Autodesk Inventor part; units mm, degrees
ref_plane "YZ Plane" through (0, 0, 0) normal (1, 0, 0) x (0, 1, 0)
ref_plane "XZ Plane" through (0, 0, 0) normal (0, 1, 0) x (-1, 0, 0)
ref_plane "XY Plane" through (0, 0, 0) normal (0, 0, 1) x (1, 0, 0)
sketch "Sketch1" plane through (0, 0, 0) normal (0, 0, 1) x (1, 0, 0)
  line L0 (0, 4.0132) -> (0, -0.9652)
  line L1 (-1.524, 0) -> (9.144, 0)
  line L2 (7.62, 0) -> (0, 0)
  line L3 (0, 0) -> (0, 0.762)
  line L4 (0, 0.762) -> (7.62, 0.762)
  line L5 (7.62, 0.762) -> (7.62, 0)
  line L6 (0, 0.762) -> (0.762, 0.762)
  line L7 (0.762, 0.762) -> (0.762, 3.302)
  line L8 (0.762, 3.302) -> (0, 3.302)
  line L9 (0, 3.302) -> (0, 0.762)
  line L10 (6.096, -0.254) -> (7.62, -0.254)
  line L11 (7.62, -0.254) -> (7.62, 1.016)
  line L12 (7.62, 1.016) -> (6.096, 1.016)
  line L13 (6.096, 1.016) -> (6.096, -0.254)
  line L14 (6.096, -0.254) -> (7.62, 1.016) construction
  line L15 (7.62, -0.254) -> (6.096, 1.016) construction
  line L16 (0, 0.381) -> (7.62, 0.381) construction
  point P0 (6.858, 0.381)
  dimension "d0" = 0.762
  dimension "d1" = 0.762
  dimension "d2" = 3.302
  dimension "d4" = 1.27
  dimension "d5" = 1.524
  dimension "d6" = 6.858
  dimension "d7" = 0
extrude "Extrusion1" add sketch "Sketch1" along normal mid plane 1.016 contours L8 L7 L4 L0 | L4 L13 L1 L0 | L13 L4 L5 L1
sketch "Sketch2" plane through (0.762, 0.762, 0.508) normal (0, 1, 0) x (1, 0, 0)
  line L0 (-0.762, 1.5748) -> (-0.762, -0.5588)
  line L1 (8.382, 0.508) -> (-2.286, 0.508)
  line L2 (6.858, 1.016) -> (6.858, 0)
  circle A0 centre (6.096, 0.508) radius 0.762
  line L3 (0, 1.016) -> (6.858, 1.016)
  line L4 (6.858, 0) -> (0, 0)
  line L5 (6.664, 0) -> (6.858, 0)
  line L6 (6.858, 0) -> (6.858, 1.016)
  line L7 (6.858, 1.016) -> (6.664, 1.016)
  line L8 (5.334, -0.2504) -> (6.0218, -0.2504)
  line L9 (6.0218, -0.2504) -> (6.0218, 1.2664)
  line L10 (6.0218, 1.2664) -> (5.334, 1.2664)
  line L11 (5.334, 1.2664) -> (5.334, -0.2504)
  line L12 (5.334, -0.2504) -> (6.0218, 1.2664) construction
  line L13 (6.0218, -0.2504) -> (5.334, 1.2664) construction
  point P0 (-0.762, 0.508)
  point P1 (5.6779, 0.508)
  dimension "d10" = 1.524
  dimension "d30" = 6.096
extrude "Extrusion2" add sketch "Sketch2" against normal blind 1.016 and the other way blind 0.254 contours A0 L4 L9 L1 | L1 L9 L3 A0 | L9 L4 A0 L1 | L1 A0 L3 L9 | L3 L9 A0 | A0 L9 L4 | L11 L3 A0 | A0 L4 L11 | L9 A0 L4 | L3 A0 L9 | A0 L3 L11 L10 | L8 L11 L4 A0
extrude "Extrusion3" cut sketch "Sketch2" against normal up to next contours A0 L3 L2 | L2 L4 A0
hole "Hole1" at (6.858, 1.016, 0) direction (0, -1, 0) diameter 0.508 end through all
fillet "Fillet2" radius 0.254 2 edges at (0.762, 0.762, 0) (0, 0, 0)
fillet "Fillet3" radius 0.127 2 edges at (6.096, 0.381, 0.508) (6.096, 0.381, -0.508)
fillet "Fillet4" radius 0.127 2 edges at (0, 3.302, 0) (0.762, 3.302, 0)
properties part number "J007872 GRIN LENS HOLDER 0_5MM DIA Rev -" material "STAINLESS STEEL, 316"
The model under review builds one solid part; all positions refer to its coordinate system, in mm. A direction names the side the tool comes from. Coordinates: 2 decimals unless noted, no trailing zeros. Loops run counter-clockwise (first coordinate to the right, second up) from the corner with the lowest first, then second, coordinate; pieces in that order, holes last.
(1) Insertion check: P1, Ø1, axis at x = 5.5, y = 2.5, coming from the -Z side. The pin has a flat end and moves straight along its axis. Give the tip position at first contact, or say it passes through.
Determined:
P1: passes through
(2) Consider section A-A, the plane x = 5.5. Give the boundary of the cut face in (y, z), plus the area to 3 significant figures.
Determined:
outline: (0, -0.51) - (0.76, -0.51) - (0.76, 0.51) - (0, 0.51) - close
area: 0.774 mm2
(3) Tool access review of faces 1 (the flat face through (0, 2, 0)), 2 (the flat face through (1.9, 0.4, 0.508)), 3 (the flat face through (1.9, 0.4, -0.508)), 4 (the flat face through (0.762, 2, 0)): name each direction out of +Z, -Z, +X, -X, +Y, -Y from which nothing blocks a thin tool from reaching the whole face with its end or side.
Determined:
face 1: +Z, -Z, -X, +Y, -Y
face 2: +Z, -X, +Y, -Y
face 3: -Z, -X, +Y, -Y
face 4: +Z, -Z, +X, +Y
(4) Wall thickness on L1, parallel to X at y = 0.6, z = 0; L2, parallel to Y at x = 5.5, z = 0.15: over which ranges is each line inside the solid? List them lowest first.
Determined:
L1: x = 0 to 6.6, 7.11 to 7.62
L2: y = 0 to 0.76
